from build123d import *

# Parameters (mm, degrees)
F1_DEPTH = 50.8
F2_W     = 6.35
F2_H     = 19.05
F3_DEPTH = 6.35


with BuildPart() as f1:
    # F0 (on Top) → F1 (new body)
    with BuildSketch(Plane.XY):
        with BuildLine():
            Line((63.5, 76.2), (-63.5, 76.2))
            ThreePointArc((-63.5, 76.2), (-72.480256, 72.480256), (-76.2, 63.5))
            Line((-76.2, 63.5), (-76.2, -63.5))
            ThreePointArc((-76.2, -63.5), (-72.480256, -72.480256), (-63.5, -76.2))
            Line((-63.5, -76.2), (63.5, -76.2))
            ThreePointArc((63.5, -76.2), (72.480256, -72.480256), (76.2, -63.5))
            Line((76.2, -63.5), (76.2, 63.5))
            ThreePointArc((76.2, 63.5), (72.480256, 72.480256), (63.5, 76.2))
        make_face()
        with BuildLine():
            ThreePointArc((-69.85, 57.15), (-66.130256, 66.130256), (-57.15, 69.85))
            Line((-57.15, 69.85), (0, 69.85))
            Line((0, 69.85), (57.15, 69.85))
            ThreePointArc((57.15, 69.85), (66.130256, 66.130256), (69.85, 57.15))
            Line((69.85, 57.15), (69.85, 0))
            Line((69.85, 0), (69.85, -57.15))
            ThreePointArc((69.85, -57.15), (66.130256, -66.130256), (57.15, -69.85))
            Line((57.15, -69.85), (0, -69.85))
            Line((0, -69.85), (-57.15, -69.85))
            ThreePointArc((-57.15, -69.85), (-66.130256, -66.130256), (-69.85, -57.15))
            Line((-69.85, -57.15), (-69.85, 0))
            Line((-69.85, 0), (-69.85, 57.15))
        make_face(mode=Mode.SUBTRACT)
    extrude(amount=-F1_DEPTH)

    # F2 (on face) → F3 (cut)
    with BuildSketch(Plane.XZ.offset(76.2)):
        with Locations((-31.75, -28.575)):
            Rectangle(F2_W, F2_H)
        with Locations((31.75, -28.575)):
            Rectangle(F2_W, F2_H)
    extrude(amount=-F3_DEPTH, mode=Mode.SUBTRACT)


solid = f1.part
For this review, take the finished solid that the model builds, in its own axes (mm). A direction names the side the tool comes from. Round coordinates to 2 decimals unless told otherwise and drop trailing zeros. Write each loop counter-clockwise with the first axis right and the second up, starting at its lowest first coordinate (ties: lowest second). Pieces come first, ordered by that corner, then holes. Notation, with made-up numbers: (-26.5, 10) - (13.5, 10) arc R19 ccw to (13.5, 29) - close; hole circle Ø9 at (14, -22.5). An arc over 180 degrees is marked (long way). Write item = value, one per line. Start each with the question number.
1. Consider section A-A on y = -13.5. State the section outline as (x, z) points, plus the area to 3 significant figures.
2. Consider section D-D on z = -12.5. State the section outline as (x, y) points, plus the area to 3 significant figures.
3. For pin 1 Ø1.9 at (y, z) = (-71.5, -24.5) entering from -X; pin 2 Ø3 at (x, y) = (-30.5, -74) entering from +Z; pin 3 Ø3 at (y, z) = (-73, -27.5) entering from -X; pin 4 Ø5 at (y, z) = (-72, -31.5) entering from +X, all flat-tipped, find the tip position at first contact; note any pin that passes through.
4. Wall thickness on L1, parallel to Y at x = -17.5, z = -36: over which ranges is the line inside the solid? List them lowest first.
5. Draft analysis for pull direction Z (two halves, no side actions). For faces 1 (the face through (-6, -73, -50.8)), 2 (the face through (32, -73, -19.05)), 3 (the face through (-66.03, -66.23, -25.04)), state which applies: released by +Z, released by -Z, zero draft, split by the parting line, or undercut.
6. Consider section B-B on z = -32.5. State the section outline as (x, y) points (3 decimals).
7. For faces 4 (the face through (-32, -73, -38.1)), 5 (the face through (69.85, 1, -25)), 6 (the face through (-1, -76.2, -25)), list the 3-axis set-ups (+Z, -Z, +X, -X, +Y, -Y) from which the entire face can be reached by the end or side of a thin tool; tool diameter is ignored.
Evaluation:
q1.outline = (-76.2, -50.8) - (-69.85, -50.8) - (-69.85, 0) - (-76.2, 0) - close; (69.85, -50.8) - (76.2, -50.8) - (76.2, 0) - (69.85, 0) - close
q1.area = 645 mm2
q2.outline = (-76.2, -63.5) arc R12.7 ccw to (-63.5, -76.2) - (63.5, -76.2) arc R12.7 ccw to (76.2, -63.5) - (76.2, 63.5) arc R12.7 ccw to (63.5, 76.2) - (-63.5, 76.2) arc R12.7 ccw to (-76.2, 63.5) - close; hole (-69.85, -57.15) arc R12.7 ccw to (-57.15, -69.85) - (57.15, -69.85) arc R12.7 ccw to (69.85, -57.15) - (69.85, 57.15) arc R12.7 ccw to (57.15, 69.85) - (-57.15, 69.85) arc R12.7 ccw to (-69.85, 57.15) - close
q2.area = 3,710 mm2
q3.pin_1 = -74.06
q3.pin_2 = 0
q3.pin_3 = -73.36
q3.pin_4 = 74.69
q4.L1 = -76.2 to -69.85, 69.85 to 76.2
q5.face_1 = released by -Z
q5.face_2 = undercut
q5.face_3 = zero draft
q6.outline = (-76.2, -63.5) arc R12.7 ccw to (-63.5, -76.2) - (-34.925, -76.2) - (-34.925, -69.85) - (-57.15, -69.85) arc R12.7 cw to (-69.85, -57.15) - (-69.85, 57.15) arc R12.7 cw to (-57.15, 69.85) - (57.15, 69.85) arc R12.7 cw to (69.85, 57.15) - (69.85, -57.15) arc R12.7 cw to (57.15, -69.85) - (34.925, -69.85) - (34.925, -76.2) - (63.5, -76.2) arc R12.7 ccw to (76.2, -63.5) - (76.2, 63.5) arc R12.7 ccw to (63.5, 76.2) - (-63.5, 76.2) arc R12.7 ccw to (-76.2, 63.5) - close; (-28.575, -76.2) - (28.575, -76.2) - (28.575, -69.85) - (-28.575, -69.85) - close
q7.face_4 = -Y
q7.face_5 = +Z, -Z
q7.face_6 = +Z, -Z, +X, -X, -Y
